Part model, mm, in its own coordinate system. Face numbers are marked on the shaded views. A direction names the side the tool comes from. Round coordinates to 2 decimals unless told otherwise and drop trailing zeros. Order: outer loops, then holes, each group sorted by start corner. A loop starts at its lowest first (then second) coordinate and runs counter-clockwise, first axis right, second up. Notation, with made-up numbers: M 41,87.25 L 60,87.25 A26 ccw 60,113.25 Z; hole C 12.25,-35.75 d9. An arc over 180 degrees is marked long. Write each question's results on one line, items separated by ' | '. Start each with the question number.
1. Band-saw the part on B-B, the plane y = -2.75. List the corners of the cut face in (x, z).
2. Band-saw the part on D-D, the plane x = -1. List the corners of the cut face in (y, z), then the cut area to 3 significant figures.
3. Band-saw the part on A-A, the plane z = 13.5. List the corners of the cut face in (x, y).
4. Which spindle directions (+Z, -Z, +X, -X, +Y, -Y) get a long thin tool onto all of the face, cutting with end or side? Do the marked faces 1, 2 and 3. Say none if no direction does.
5. Band-saw the part on C-C, the plane z = 7.5. List the corners of the cut face in (x, y), then the cut area to 3 significant figures.
6. Probe L1, parallel to X at y = 1.75, z = 17.5; L2, parallel to Y at x = -22.15, z = 13.5; L3, parallel to Y at x = -8, z = -6.25. List the from-to ranges inside material, lowest first. Write a range as [from, to].
7. Two-plate mould, pull along X, no slides. Class the marked faces 4, 5 and 6: +X half, -X half, draft (parallel to the pull), parting line (faces both ways), or undercut.
8. Drop flat-ended pins along their axis: pin 1 Ø6 at (x, y) = (18, -5) entering from +Z; pin 2 Ø4 at (x, y) = (6.5, 1) entering from +Z; pin 3 Ø3.5 at (x, y) = (-2, 1) entering from -Z. Give the stop position or say it passes through.
```python
from build123d import *

# Parameters (mm, degrees)
BOSS_EXTRUDE1_DEPTH = 3
SKETCH3_W           = 4.5
SKETCH3_H           = 15
BOSS_EXTRUDE3_DEPTH = 7
CUT_EXTRUDE1_REACH  = 55.313
SKETCH4_R           = 1.7
FILLET2_R           = 5
FILLET3_R           = 2


with BuildPart() as part:
    # Sketch1 → Boss-Extrude1 (new body)
    with BuildSketch(Plane(origin=(0, 0, 0), x_dir=(1, 0, 0), z_dir=(0, 1, 0))):
        Polygon((-5, 0), (5, 0), (5, 8), (10, 8), (24.25, 0), (24.25, -21), (19.75, -21), (19.75, -4), (-19.75, -4), (-19.75, -21), (-24.25, -21), (-24.25, 0), (-10, 8), (-5, 8), align=None)
    extrude(amount=BOSS_EXTRUDE1_DEPTH)

    # Sketch3 → Boss-Extrude3 (add)
    with BuildSketch(Plane.XZ):
        with Locations((22, 13.5)):
            Rectangle(SKETCH3_W, SKETCH3_H)
    boss_extrude3 = extrude(amount=BOSS_EXTRUDE3_DEPTH)

    # Sketch4 → Cut-Extrude1 (cut, up to next)
    with BuildSketch(Plane(origin=(24.25, 0, 0), x_dir=(0, 0, -1), z_dir=(1, 0, 0)), mode=Mode.PRIVATE) as cut_extrude1_sk1:
        with Locations((-13.5, -2)):
            Circle(SKETCH4_R)
    cut_extrude1_tool1 = extrude(cut_extrude1_sk1.sketch, amount=-CUT_EXTRUDE1_REACH, mode=Mode.PRIVATE) & part.part
    cut_extrude1 = cut_extrude1_tool1.solids().sort_by_distance((24.25, -2, 13.5))[0]
    add(cut_extrude1, mode=Mode.SUBTRACT)

    # Mirror2: Boss-Extrude3, Cut-Extrude1 across plane
    add(boss_extrude3.mirror(Plane(origin=(0, 0, 0), x_dir=(0, 0, 1), z_dir=(1, 0, 0))))
    add(cut_extrude1.mirror(Plane(origin=(0, 0, 0), x_dir=(0, 0, 1), z_dir=(1, 0, 0))), mode=Mode.SUBTRACT)

    # Fillet2
    fillet2_edges = [part.edges().sort_by_distance(p)[0] for p in [
        (22, -7, 6),
        (22, -7, 21),
        (22, 3, 21),
        (-22, -7, 6),
        (-22, -7, 21),
        (-22, 3, 21),
    ]]
    fillet(fillet2_edges, radius=FILLET2_R - 0.0001)  # a hair under: the kernel refuses the full size

    # Fillet3
    fillet3_edges = [part.edges().sort_by_distance(p)[0] for p in [
        (22, 0, 6),
        (-22, 0, 6),
    ]]
    fillet(fillet3_edges, radius=FILLET3_R)


solid = part.part
```
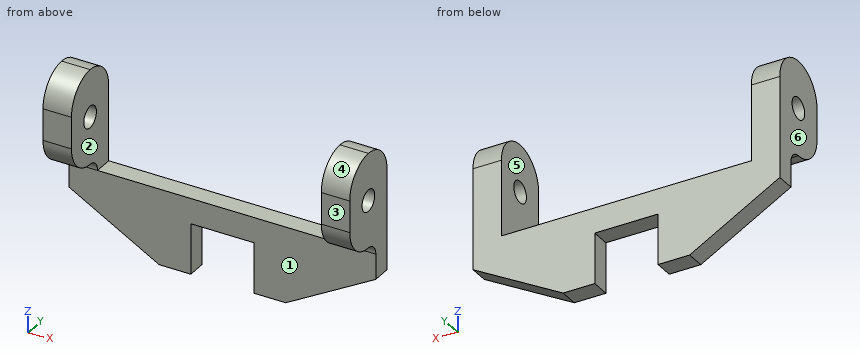
Solution:
1) outline: M -24.25,6.06 L -19.75,6.06 L -19.75,11.97 L -24.25,11.97 Z; M -24.25,15.03 L -19.75,15.03 L -19.75,20.94 L -24.25,20.94 Z; M 19.75,6.06 L 24.25,6.06 L 24.25,11.97 L 19.75,11.97 Z; M 19.75,15.03 L 24.25,15.03 L 24.25,20.94 L 19.75,20.94 Z
2) outline: M 0,0 L 3,0 L 3,4 L 0,4 Z | area: 12.0 mm^2
3) outline: M -24.25,-7 L -19.75,-7 L -19.75,-3.7 L -24.25,-3.7 Z; M -24.25,-0.3 L -19.75,-0.3 L -19.75,3 L -24.25,3 Z; M 19.75,-7 L 24.25,-7 L 24.25,-3.7 L 19.75,-3.7 Z; M 19.75,-0.3 L 24.25,-0.3 L 24.25,3 L 19.75,3 Z
4) face 1: -Z, +X, -X, -Y | face 2: +Z, +Y, -Y | face 3: +Z, -Z, +X, -X, -Y
5) outline: M -24.25,-5.57 L -19.75,-5.57 L -19.75,3 L -24.25,3 Z; M 19.75,-5.57 L 24.25,-5.57 L 24.25,3 L 19.75,3 Z | area: 77.1 mm^2
6) L1: [-24.25, -19.75], [19.75, 24.25] | L2: [-7, -3.7], [-0.3, 3] | L3: [0, 3]
7) face 4: draft | face 5: undercut | face 6: -X half
8) pin 1: z = 20.97 | pin 2: z = 4 | pin 3: z = 0
